Verification items for the finished model (mm, model axes). A direction names the side the tool comes from. Coordinates: 2 decimals unless noted, no trailing zeros. Order: outer loops, then holes, each group sorted by start corner. A loop starts at its lowest first (then second) coordinate and runs counter-clockwise, first axis right, second up. Notation, with made-up numbers: M 87.25,58 L 124.25,58 A3 cw 124.25,63 Z; hole C -13.5,87.25 d5. An arc over 180 degrees is marked long. Return JSON: item names as keys, results as strings.
```python
from build123d import *

# Parameters (mm, degrees)
CUT_EXTRUDE_1_DEPTH = 3
FILLET_1_R          = 1
CHAMFER_1_SIZE      = 0.5


with BuildPart() as part:
    # 草图1 → 旋转1 (revolve)
    with BuildSketch(Plane.XY):
        Polygon((0, 0), (0, 5), (4.5, 5), (4.5, 3), (16.5, 3), (16.5, 2.5), (26.5, 2.5), (26.5, 0), align=None)
    revolve(axis=Axis((0, 0, 0), (1, 0, 0)))

    # 草图2 → 切除-拉伸1 (cut)
    with BuildSketch(Plane.ZY):
        Polygon((0, 1.732050808), (-1.5, 0.866025404), (-1.5, -0.866025404), (0, -1.732050808), (1.5, -0.866025404), (1.5, 0.866025404), align=None)
    extrude(amount=-CUT_EXTRUDE_1_DEPTH, mode=Mode.SUBTRACT)

    # 圆角1
    fillet_1_edges = [part.edges().sort_by_distance(p)[0] for p in [
        (0, -5, 0),
    ]]
    fillet(fillet_1_edges, radius=FILLET_1_R)

    # 倒角1
    chamfer_1_edges = [part.edges().sort_by_distance(p)[0] for p in [
        (26.5, -2.5, 0),
    ]]
    chamfer(chamfer_1_edges, length=CHAMFER_1_SIZE)


solid = part.part
```
Q1. Material ranges on line 1 along Z through (x, y) = (2, 0.25); line 2 along X through (y, z) = (-3.25, -1.75); line 3 along X through (y, z) = (-0.75, 0.75), recorded low to high.
Values:
{"line 1": "-4.99 to -1.5, 1.5 to 4.99", "line 2": "0 to 4.5", "line 3": "3 to 26.5"}
Q2. Cross-section at B-B, the plane x = 15.75. Record the boundary of the cut face in (y, z), and give its area (3 significant figures).
Values:
{"outline": "C 0,0 d6", "area": "28.3 mm^2"}
Q3. Cross-section at A-A, the plane y = 0. Record the boundary of the cut face in (x, z).
Values:
{"outline": "M 0,-4 A1 ccw 1,-5 L 4.5,-5 L 4.5,-3 L 16.5,-3 L 16.5,-2.5 L 26,-2.5 L 26.5,-2 L 26.5,2 L 26,2.5 L 16.5,2.5 L 16.5,3 L 4.5,3 L 4.5,5 L 1,5 A1 ccw 0,4 L 0,1.5 L 3,1.5 L 3,-1.5 L 0,-1.5 Z"}
Q4. Draft check along Y on faces 4 (the face through (1.479, -1.293, -0.76)), 5 (the face through (16.5, -2, 2)), 6 (the face through (21.32, -0.54, -2.44)). Enter one of: pulls with the +Y half, pulls with the -Y half, needs draft (parallel to the pull), parting line crosses it, or undercut.
Values:
{"face 4": "undercut", "face 5": "needs draft", "face 6": "parting line crosses it"}
Q5. Go/stop test with flat-tipped pins: pin 1 (0.9 mm diameter, centred on y = -0.5, z = 0.5, fed in from -X); pin 2 (1 mm diameter, centred on x = 10, z = 2.5, fed in from -Y); pin 3 (5 mm diameter, centred on x = 17, z = -1, fed in from -Y). Record where each tip stops, or that it passes through.
Values:
{"pin 1": "x = 3", "pin 2": "y = -2.24", "pin 3": "y = -3"}
Q6. Cross-section at C-C, the plane x = 4. Record the boundary of the cut face in (y, z), and give its area (3 significant figures).
Values:
{"outline": "C 0,0 d10", "area": "78.5 mm^2"}
Q7. Tool access check on faces 1 (the face through (2.77, -1.08, -4.88)), 2 (the face through (11, -3, 0)), 3 (the face through (1.479, 1.305, -0.74)). Record the directions out of +Z, -Z, +X, -X, +Y, -Y that give a thin tool (end or side, any length) a straight path to the whole face; none if there is none.
Values:
{"face 1": "+X, -X", "face 2": "+X", "face 3": "-X"}
